from build123d import *

# Parameters (mm, degrees)
EXTRUDE1_DEPTH        = 12.7
SKETCH2_R             = 3.96875
CUT_EXTRUDE1_DEPTH    = 172.656838198
SKETCH3_W             = 12.7
SKETCH3_H             = 12.7
EXTRUDE2_DEPTH        = 172.656838198
SKETCH4_W             = 105.983052191
SKETCH4_H             = 75.202262717
EXTRUDE3_DEPTH        = 172.656838198
CROQUIS1_W            = 8.075015689
CROQUIS1_H            = 80
CORTAR_EXTRUIR1_DEPTH = 12.7


with BuildPart() as part:
    # Sketch1 → Extrude1 (new body)
    with BuildSketch(Plane.XY):
        with BuildLine():
            Line((-95.25, 12.7), (-53.975, 12.7))
            Line((-53.975, 12.7), (-53.975, 0))
            Line((-53.975, 0), (-34.925, 0))
            Line((-34.925, 0), (-34.925, 12.7))
            Line((-34.925, 12.7), (34.925, 12.7))
            Line((34.925, 12.7), (34.925, 0))
            Line((34.925, 0), (53.975, 0))
            Line((53.975, 0), (53.975, 12.7))
            Line((53.975, 12.7), (95.25, 12.7))
            Line((95.25, 12.7), (95.25, 142.24))
            Line((95.25, 142.24), (63.5, 142.24))
            ThreePointArc((63.5, 142.24), (0, 78.74), (-63.5, 142.24))
            Line((-63.5, 142.24), (-95.25, 142.24))
            Line((-95.25, 142.24), (-95.25, 12.7))
        make_face()
    extrude(amount=EXTRUDE1_DEPTH)

    # Sketch2 → Cut-Extrude1 (cut, through all)
    with BuildSketch(Plane.XY.offset(12.7)):
        with Locations((44.45, 66.04)):
            Circle(SKETCH2_R)
    extrude(amount=-CUT_EXTRUDE1_DEPTH, mode=Mode.SUBTRACT)

    # Sketch3 → Extrude2 (cut, through all)
    with BuildSketch(Plane.XY.offset(12.7)):
        with Locations((-88.9, 19.05)):
            Rectangle(SKETCH3_W, SKETCH3_H)
    extrude(amount=-EXTRUDE2_DEPTH, mode=Mode.SUBTRACT)

    # Sketch4 → Extrude3 (cut, through all)
    with BuildSketch(Plane.XY.offset(12.7)):
        with Locations((52.991526096, 116.341131359)):
            Rectangle(SKETCH4_W, SKETCH4_H)
    extrude(amount=-EXTRUDE3_DEPTH, mode=Mode.SUBTRACT)

    # Croquis1 → Cortar-Extruir1 (cut)
    with BuildSketch(Plane.XY.offset(12.7)):
        with Locations((-91.212492156, 76.84)):
            Rectangle(CROQUIS1_W, CROQUIS1_H)
    extrude(amount=-CORTAR_EXTRUIR1_DEPTH, mode=Mode.SUBTRACT)


solid = part.part
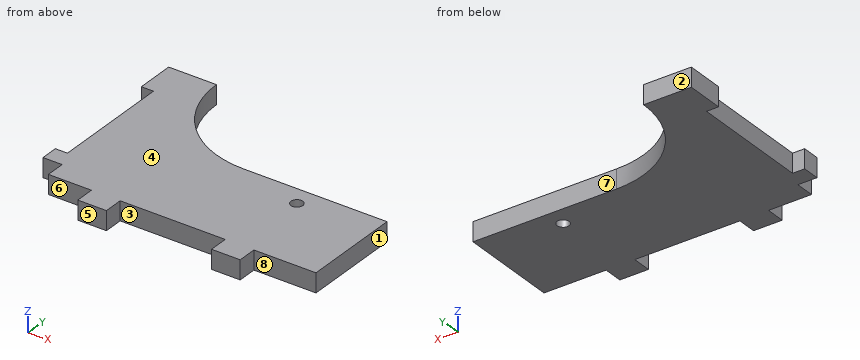
Work out the finished part from the listing and answer in its coordinate system (mm). Face numbers are marked on the shaded views. A direction names the side the tool comes from. Round coordinates to 2 decimals unless told otherwise and drop trailing zeros. Write each loop counter-clockwise with the first axis right and the second up, starting at its lowest first coordinate (ties: lowest second). Pieces come first, ordered by that corner, then holes. Notation, with made-up numbers: M 86,34 L 121,34 A11 cw 121,47 Z; hole C 16.5,82.5 d8. An arc over 180 degrees is marked long. Use a Markdown table: item, result.
1) Consider line 1 (Y direction, x = 44.45, z = 7.25); line 2 (X direction, y = 41, z = 6.75); line 3 (Y direction, x = 21, z = 9.5). Determine where each line is inside the solid, lowest interval first. Write a range as [from, to].
Taken from the geometry:
| item | result |
|---|---|
| line 1 | y = [0, 62.07], [70.01, 78.74] |
| line 2 | x = [-87.17, 95.25] |
| line 3 | y = [12.7, 78.74] |
2) Flat-ended cylindrical pins translate along their axes: pin 1 (6.5 mm diameter, centred on y = 5, z = 7, fed in from -X) (3 decimals); pin 2 (7 mm diameter, centred on x = 44.45, y = 66.04, fed in from -Z); pin 3 (4 mm diameter, centred on y = 87, z = 3.5, fed in from -X) (3 decimals); pin 4 (3 mm diameter, centred on x = 25, z = 3.5, fed in from +Y). Find the tip coordinate at first contact, or state that the pin passes through.
Taken from the geometry:
| item | result |
|---|---|
| pin 1 | stops at x = -53.975 |
| pin 2 | passes through |
| pin 3 | stops at x = -87.175 |
| pin 4 | stops at y = 78.74 |
3) Determine the mould class of the marked faces 1, 2 and 3 for opening direction X: pulls with the +X half, pulls with the -X half, needs draft (parallel to the pull), parting line crosses it, or undercut.
Taken from the geometry:
| item | result |
|---|---|
| face 1 | pulls with the +X half |
| face 2 | needs draft |
| face 3 | undercut |
4) The part is cut by section B-B on y = 66.04. Give the vertices of the cut face in (x, z), plus the area to 3 significant figures.
Taken from the geometry:
| item | result |
|---|---|
| outline | M -87.17,0 L 40.48,0 L 40.48,12.7 L -87.17,12.7 Z; M 48.42,0 L 95.25,0 L 95.25,12.7 L 48.42,12.7 Z |
| area | 2,220 mm2 |
5) Which of the six approach directions +Z, -Z, +X, -X, +Y, -Y give full straight-line access (tool end or side, diameter ignored) to the marked faces 4, 5, 6, 7 and 8?
Taken from the geometry:
| item | result |
|---|---|
| face 4 | +Z, +X, -X, +Y, -Y |
| face 5 | +Z, -Z, +X, -X, -Y |
| face 6 | +Z, -Z, -X, -Y |
| face 7 | +Z, -Z, +X, +Y |
| face 8 | +Z, -Z, +X, -Y |
6) The part is cut by section D-D on x = 74.5. Give the vertices of the cut face in (y, z), plus the area to 3 significant figures.
Taken from the geometry:
| item | result |
|---|---|
| outline | M 12.7,0 L 78.74,0 L 78.74,12.7 L 12.7,12.7 Z |
| area | 839 mm2 |
7) The part is cut by section A-A on x = 44.45. Give the vertices of the cut face in (y, z).
Taken from the geometry:
| item | result |
|---|---|
| outline | M 0,0 L 62.07,0 L 62.07,12.7 L 0,12.7 Z; M 70.01,0 L 78.74,0 L 78.74,12.7 L 70.01,12.7 Z |
